from build123d import *

# Parameters (mm, degrees)
SKETCH_2_R          = 3
EXTRUDE_1_DEPTH     = 6
SKETCH_3_R          = 5
EXTRUDE_2_DEPTH     = 29.58
SKETCH_4_R          = 2.55
CUT_EXTRUDE_1_DEPTH = 55.029865815
CHAMFER_1_SIZE      = 1


with BuildPart() as part:
    # 草图2 → 凸台-拉伸1 (new body)
    with BuildSketch(Plane.XY):
        with BuildLine():
            Line((26.49133381, -23.443703305), (-3.03527618, -15.532072003))
            ThreePointArc((-3.03527618, -15.532072003), (-5.173413361, -14.103414414), (-6, -11.668368698))
            Line((-6, -11.668368698), (-6, 2))
            ThreePointArc((-6, 2), (-4.828427125, 4.828427125), (-2, 6))
            Line((-2, 6), (39.5, 6))
            Line((39.5, 6), (39.5, -23.58))
            Line((39.5, -23.58), (27.52660999, -23.58))
            ThreePointArc((27.52660999, -23.58), (27.004505221, -23.545779445), (26.49133381, -23.443703305))
        make_face()
        Circle(SKETCH_2_R, mode=Mode.SUBTRACT)
        with Locations((20, 0)):
            Circle(SKETCH_2_R, mode=Mode.SUBTRACT)
        with Locations((20, -12.5)):
            Circle(SKETCH_2_R, mode=Mode.SUBTRACT)
    extrude(amount=EXTRUDE_1_DEPTH)

    # 草图3 → 凸台-拉伸2 (add, through all)
    with BuildSketch(Plane(origin=(0, 6, 0), x_dir=(1, 0, 0), z_dir=(0, 1, 0))):
        with Locations((39.5, -3)):
            Circle(SKETCH_3_R)
    extrude(amount=-EXTRUDE_2_DEPTH)

    # 草图4 → 切除-拉伸1 (cut, through all)
    with BuildSketch(Plane(origin=(0, 6, 0), x_dir=(1, 0, 0), z_dir=(0, 1, 0))):
        with Locations(Location((39.5, -3, 0), (0, 0, 270))):
            Circle(SKETCH_4_R)
    extrude(amount=-CUT_EXTRUDE_1_DEPTH, mode=Mode.SUBTRACT)

    # 倒角1
    chamfer_1_edges = [part.edges().sort_by_distance(p)[0] for p in [
        (31.513304995, -23.58, 0),
        (27.004505221, -23.545779445, 0),
        (-4.828427125, 4.828427125, 6),
        (-3, 0, 0),
        (-3, 0, 6),
        (-6, -4.834184349, 6),
        (17, 0, 0),
        (17, 0, 6),
        (-5.173413361, -14.103414414, 6),
        (17, -12.5, 0),
        (17, -12.5, 6),
        (11.728028815, -19.487887654, 6),
        (16.75, 6, 0),
        (16.75, 6, 6),
        (44.5, -23.58, 3),
        (44.5, 6, 3),
        (27.004505221, -23.545779445, 6),
        (39.5, 6, 0.45),
        (11.728028815, -19.487887654, 0),
        (31.513304995, -23.58, 6),
        (-5.173413361, -14.103414414, 0),
        (-6, -4.834184349, 0),
        (-4.828427125, 4.828427125, 0),
    ]]
    chamfer(chamfer_1_edges, length=CHAMFER_1_SIZE)


solid = part.part
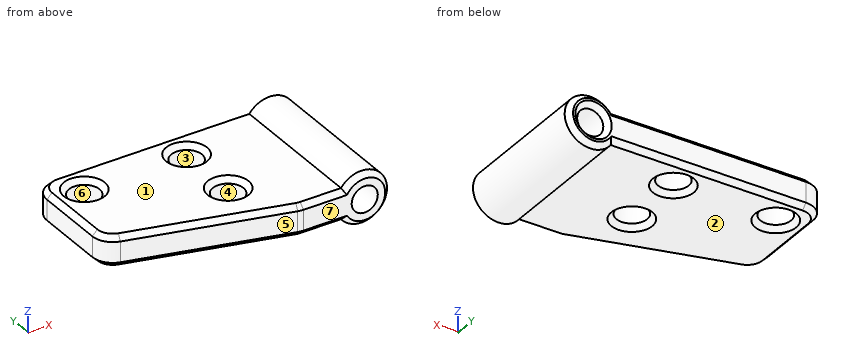
CAD build for the part. Positions are in the model's coordinates, mm. Face numbers are marked on the shaded views. A direction names the side the tool comes from. Round coordinates to 2 decimals unless told otherwise and drop trailing zeros. Write each loop counter-clockwise with the first axis right and the second up, starting at its lowest first coordinate (ties: lowest second). Pieces come first, ordered by that corner, then holes.
(1) 3-axis set-ups, long thin cutter, end or side, ignore diameter. For the marked faces 1, 2 and 3: which of +Z, -Z, +X, -X, +Y, -Y reach the whole face in a straight line?
(2) Mould opens along X. For the marked faces 4, 5, 6 and 7 say: pulls with the +X half, pulls with the -X half, needs draft (parallel to the pull), parting line crosses it, or undercut.
(3) Probe line 1 along X through (y, z) = (-8, 3); line 2 along X through (y, z) = (-13.25, 3.5); line 3 along Z through (x, y) = (27, -16.5). List the from-to ranges inside material, lowest first.
(4) Slice it at A-A, the plane z = 3. Write the cut outline in (x, y).
(5) Slice it at B-B, the plane y = 0. Write the cut outline in (x, z).
(6) Slice it at D-D, the plane y = -7.25. Write the cut outline in (x, z).
(7) Drop flat-ended pins along their axis: P1, Ø12, axis at x = 32.5, y = -15.5, coming from the -Z side; P2, Ø8.5, axis at x = 13, y = -4.5, coming from the -Z side; P3, Ø3.5, axis at x = 20, y = -12.5, coming from the +Z side; P4, Ø1, axis at y = -8.5, z = 0.5, coming from the +X side. Give the stop position or say it passes through.
(8) Slice it at C-C, the plane x = 39.5. Write the cut outline in (y, z), and give its area (3 significant figures).
From the geometry:
1. face 1: +Z, -X, +Y, -Y
1. face 2: -Z, -X, +Y, -Y
1. face 3: +Z, -Z
2. face 4: undercut
2. face 5: pulls with the -X half
2. face 6: undercut
2. face 7: needs draft
3. line 1: x = -6 to 36.95, 42.05 to 44.5
3. line 2: x = -5.67 to 17.1, 22.9 to 37, 42 to 44.47
3. line 3: z = 0 to 6
4. outline: (-6, -11.67) arc R4 ccw to (-3.04, -15.53) - (26.49, -23.44) arc R4 ccw to (27.53, -23.58) - (36.95, -23.58) - (36.95, 5) - (35.95, 6) - (-2, 6) arc R4 ccw to (-6, 2) - close; (42.05, -23.58) - (43.5, -23.58) - (44.5, -22.58) - (44.5, 5) - (43.5, 6) - (43.05, 6) - (42.05, 5) - close; hole circle Ø6 at (0, 0); hole circle Ø6 at (20, -12.5); hole circle Ø6 at (20, 0)
5. outline: (-6, 1) - (-5, 0) - (-4, 0) - (-3, 1) - (-3, 5) - (-4, 6) - (-5, 6) - (-6, 5) - close; (3, 1) - (4, 0) - (16, 0) - (17, 1) - (17, 5) - (16, 6) - (4, 6) - (3, 5) - close; (23, 1) - (24, 0) - (35.5, 0) arc R5 ccw (long way) to (35.5, 6) - (24, 6) - (23, 5) - close; hole circle Ø5.1 at (39.5, 3)
6. outline: (-6, 1) - (-5, 0) - (35.5, 0) arc R5 ccw (long way) to (35.5, 6) - (-5, 6) - (-6, 5) - close; hole circle Ø5.1 at (39.5, 3)
7. P1: stops at z = -1.9
7. P2: stops at z = 0
7. P3: passes through
7. P4: stops at x = 44.08
8. outline: (-23.58, -1) - (-22.58, -2) - (5, -2) - (6, -1) - (6, -0.55) - (5, 0.45) - (-23.58, 0.45) - close; (-23.58, 5.55) - (5, 5.55) - (6, 6.55) - (6, 7) - (5, 8) - (-22.58, 8) - (-23.58, 7) - close
8. area: 142 mm2
